Check sheet for the modelled part. Datum: model origin and axes. Units: mm. Face numbers are marked on the shaded views. A direction names the side the tool comes from. Give positions to 0.01 mm unless a question says otherwise; leave off trailing zeros. Loops run counter-clockwise (first coordinate to the right, second up) from the corner with the lowest first, then second, coordinate; pieces in that order, holes last. Notation, with made-up numbers: M 10.5,51 L 68.5,51 A15 ccw 68.5,59 Z; hole C -10.75,-33 d3. An arc over 180 degrees is marked long. Use one line per item in the form item = value.
from build123d import *

# Parameters (mm, degrees)
SKETCH1_R           = 190.5
SKETCH1_R_2         = 127
BOSS_EXTRUDE1_DEPTH = 50.8
CUT_EXTRUDE1_DEPTH  = 25.4
CIRPATTERN1_COUNT   = 10
CIRPATTERN1_ANGLE   = 180


with BuildPart() as part:
    # Sketch1 → Boss-Extrude1 (new body)
    with BuildSketch(Plane.XY):
        Circle(SKETCH1_R)
        Circle(SKETCH1_R_2, mode=Mode.SUBTRACT)
    extrude(amount=BOSS_EXTRUDE1_DEPTH)

    # Sketch2 → Cut-Extrude1 (cut)
    with BuildSketch(Plane.XY.offset(50.8)):
        with BuildLine():
            Line((19.05, 152.4), (19.05, -152.4))
            ThreePointArc((19.05, -152.4), (0, -171.45), (-19.05, -152.4))
            Line((-19.05, -152.4), (-19.05, 152.4))
            ThreePointArc((-19.05, 152.4), (0, 171.45), (19.05, 152.4))
        make_face()
    cut_extrude1 = extrude(amount=-CUT_EXTRUDE1_DEPTH, mode=Mode.SUBTRACT)

    # CirPattern1: Cut-Extrude1 ×10 about axis
    cirpattern1_axis = Axis((0, 0, 0), (0, 0, 1))
    for i in range(1, CIRPATTERN1_COUNT):
        add(cut_extrude1.rotate(cirpattern1_axis, i * CIRPATTERN1_ANGLE / (CIRPATTERN1_COUNT - 1)), mode=Mode.SUBTRACT)


solid = part.part
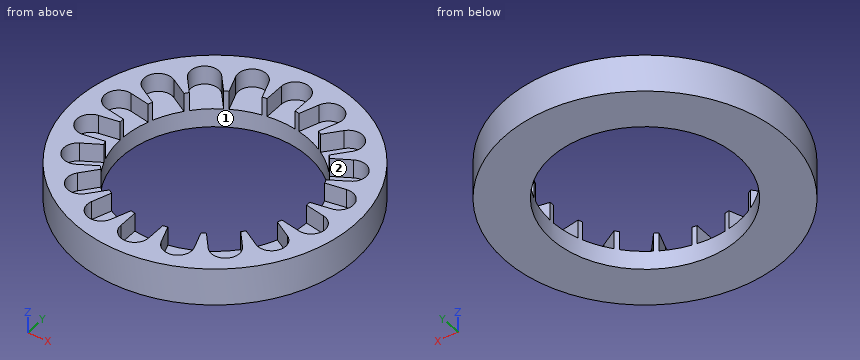
1) Scan lines: line 1 (Y direction, x = 0, z = 28.5); line 2 (Y direction, x = 0, z = 10); line 3 (X direction, y = -129.5, z = 43). Record each from-to range of solid material in increasing order.
Evaluation:
line_1 = -190.5 to -171.45, 171.45 to 190.5
line_2 = -190.5 to -127, 127 to 190.5
line_3 = -139.71 to -112.11, -83.81 to -67.41, -26.86 to -19.05, 19.05 to 26.86, 67.41 to 83.81, 112.11 to 139.71
2) Set-up check for the marked faces 1 and 2: record each of +Z, -Z, +X, -X, +Y, -Y from which the full face is reachable in a straight line by a thin tool's end or side.
Evaluation:
face_1 = +Z, -Z
face_2 = +Z
3) Section check A-A (x = 0). Record the cut outline in (y, z), then the cut area to 3 significant figures.
Evaluation:
outline = M -190.5,0 L -127,0 L -127,25.4 L -171.45,25.4 L -171.45,50.8 L -190.5,50.8 Z; M 127,0 L 190.5,0 L 190.5,50.8 L 171.45,50.8 L 171.45,25.4 L 127,25.4 Z
area = 4,190 mm^2
4) Depth check by flat-ended pin: pin 1 Ø12.5 at (x, y) = (-150.5, -30) entering from +Z; pin 2 Ø3 at (x, z) = (88, 31.5) entering from +Y; pin 3 Ø5 at (y, z) = (-33, 6) entering from -X. Enter the tip coordinate at first touch or a pass-through.
Evaluation:
pin_1 = 25.4
pin_2 = 169.73
pin_3 = -188.04
5) Section check B-B (y = -52). Record the cut outline in (x, z).
Evaluation:
outline = M -183.27,0 L -115.87,0 L -115.87,25.4 L -128.17,25.4 L -128.17,50.8 L -183.27,50.8 Z; M 115.87,0 L 183.27,0 L 183.27,50.8 L 128.17,50.8 L 128.17,25.4 L 115.87,25.4 Z
6) Section check C-C (z = 9). Record the cut outline in (x, y), then the cut area to 3 significant figures.
Evaluation:
outline = C 0,0 d381; hole C 0,0 d254
area = 63,300 mm^2
